Autodesk Fusion 360 part; units mm, degrees
sketch "Sketch1" plane through (0, 0, 0) normal (0, 0, 1) x (1, 0, 0)
  line L0 (-4.25, 7.25) -> (4.25, 7.25)
  line L1 (7.25, 4.25) -> (7.25, -4.25)
  line L2 (4.25, -7.25) -> (-4.25, -7.25)
  line L3 (-7.25, -4.25) -> (-7.25, 4.25)
  line L4 (-7.25, 7.25) -> (7.25, -7.25) construction
  line L5 (7.25, 7.25) -> (-7.25, -7.25) construction
  arc A0 (-4.25, 7.25) -> (-7.25, 4.25) centre (-4.25, 4.25) ccw
  arc A1 (-7.25, -4.25) -> (-4.25, -7.25) centre (-4.25, -4.25) ccw
  arc A2 (4.25, -7.25) -> (7.25, -4.25) centre (4.25, -4.25) ccw
  arc A3 (7.25, 4.25) -> (4.25, 7.25) centre (4.25, 4.25) ccw
  line L6 (10, 10) -> (-10, 10)
  line L7 (-15, 5) -> (-15, -5)
  line L8 (-10, -10) -> (10, -10)
  line L9 (15, -5) -> (15, 5)
  line L10 (15, 10) -> (-15, -10) construction
  line L11 (-15, 10) -> (15, -10) construction
  arc A4 (15, 5) -> (10, 10) centre (10, 5) ccw
  arc A5 (-10, 10) -> (-15, 5) centre (-10, 5) ccw
  arc A6 (-15, -5) -> (-10, -10) centre (-10, -5) ccw
  arc A7 (10, -10) -> (15, -5) centre (10, -5) ccw
  circle A8 centre (-12.5, 0) radius 1.6
  line L12 (0, 0) -> (0, 5.6259) construction
  circle A9 centre (12.5, 0) radius 1.6
  line L13 (-3, 4.4279) -> (-3, -3.4951) construction
  line L14 (6.15, 5.55) -> (-6.15, 5.55)
  line L15 (-6.15, 5.55) -> (-6.15, -5.55)
  line L16 (-6.15, -5.55) -> (6.15, -5.55)
  line L17 (6.15, -5.55) -> (6.15, 5.55)
  line L18 (6.15, 5.55) -> (-6.15, -5.55) construction
  line L19 (-6.15, 5.55) -> (6.15, -5.55) construction
  line L20 (-6.35, -5.75) -> (6.35, -5.75)
  line L21 (6.35, -5.75) -> (6.35, 5.75)
  line L22 (6.35, 5.75) -> (-6.35, 5.75)
  line L23 (-6.35, 5.75) -> (-6.35, -5.75)
  dimension "d1" = 14.5
  dimension "d2" = 14.5
  dimension "d3" = 3
  dimension "d4" = 30
  dimension "d5" = 20
  dimension "d6" = 5
  dimension "d7" = 3.2
  dimension "d17" = 12.5
  dimension "d21" = 12.3
  dimension "d22" = 11.1
  dimension "d23" = 0.2
extrude "Extrude1" add sketch "Sketch1" along normal blind 2.5 contours L0 L1 L2 L3 A0 A1 A2 A3 | L6 L7 L8 L9 A4 A5 A6 A7 | L20 L21 L22 L23
extrude "Extrude2" add sketch "Sketch1" against normal blind 11 contours L0 L1 L2 L3 A0 A1 A2 A3
Input: part model. Units: mm. Frame: model coordinates. A direction names the side the tool comes from. Give positions to 0.01 mm unless a question says otherwise; leave off trailing zeros. Order: outer loops, then holes, each group sorted by start corner. A loop starts at its lowest first (then second) coordinate and runs counter-clockwise, first axis right, second up.
Q1. Draft query along Y for faces 1 (the flat face through (0, 5.75, -5)), 2 (the flat face through (-6.35, 0, -5)), 3 (the cylindrical face through (13, 9, 1)), 4 (the flat face through (15, 0, 1)). Return one class per face: +Y half, -Y half, draft (parallel to the pull), parting line (faces both ways), or undercut.
Checked values:
face 1: undercut
face 2: undercut
face 3: +Y half
face 4: draft
Q2. Contact query for flat-ended pins moving along their axis: pin 1 Ø4 at (x, z) = (2, -4.5) entering from -Y; pin 2 Ø3.5 at (y, z) = (-1.5, -3) entering from -X; pin 3 Ø2 at (y, z) = (-1.5, -9.5) entering from +X. Output: stop coordinate, or through.
Checked values:
pin 1: stops at y = -7.25
pin 2: stops at x = -7.25
pin 3: stops at x = 7.25
Q3. Section A-A on y = 0. Output: boundary loops of the cut face in (x, z).
Checked values:
outline: (-15, 0) - (-14.1, 0) - (-14.1, 2.5) - (-15, 2.5) - close; (-10.9, 0) - (-7.25, 0) - (-7.25, -11) - (-6.35, -11) - (-6.35, 0) - (-6.15, 0) - (-6.15, 2.5) - (-10.9, 2.5) - close; (6.15, 0) - (6.35, 0) - (6.35, -11) - (7.25, -11) - (7.25, 0) - (10.9, 0) - (10.9, 2.5) - (6.15, 2.5) - close; (14.1, 0) - (15, 0) - (15, 2.5) - (14.1, 2.5) - close
Q4. Ray query, probe 1 along Y at (x, z) = (-3.5, -4.5); probe 2 along X at (y, z) = (0.25, -3.75); probe 3 along X at (y, z) = (2.75, 0.25). Return the intervals inside material, ascending.
Checked values:
probe 1: y = -7.25 to -5.75, 5.75 to 7.25
probe 2: x = -7.25 to -6.35, 6.35 to 7.25
probe 3: x = -15 to -6.15, 6.15 to 15
Q5. Set-up query: faces 5 (the flat face through (-7.25, 0, -5)), 6 (the cylindrical face through (6.39, 6.35, -5.42)), 7 (the cylindrical face through (6.35, -6.39, -5.42)). Return all of +Z, -Z, +X, -X, +Y, -Y with unobstructed straight access to the full face (end or side cutting, diameter ignored); none if empty.
Checked values:
face 5: -Z, -X, +Y, -Y
face 6: -Z, +X, +Y
face 7: -Z, +X, -Y
Q6. Section C-C on z = -8.25. Output: boundary loops of the cut face in (x, y), and give its area (3 significant figures).
Checked values:
outline: (-7.25, -4.25) arc R3 ccw to (-4.25, -7.25) - (4.25, -7.25) arc R3 ccw to (7.25, -4.25) - (7.25, 4.25) arc R3 ccw to (4.25, 7.25) - (-4.25, 7.25) arc R3 ccw to (-7.25, 4.25) - close; hole (-6.35, -5.75) - (6.35, -5.75) - (6.35, 5.75) - (-6.35, 5.75) - close
area: 56.5 mm2
Q7. Section B-B on y = -3.5. Output: boundary loops of the cut face in (x, z).
Checked values:
outline: (-15, 0) - (-7.25, 0) - (-7.25, -11) - (-6.35, -11) - (-6.35, 0) - (-6.15, 0) - (-6.15, 2.5) - (-15, 2.5) - close; (6.15, 0) - (6.35, 0) - (6.35, -11) - (7.25, -11) - (7.25, 0) - (15, 0) - (15, 2.5) - (6.15, 2.5) - close
Q8. Section D-D on x = 12.75. Output: boundary loops of the cut face in (y, z), and give its area (3 significant figures).
Checked values:
outline: (-9.18, 0) - (-1.58, 0) - (-1.58, 2.5) - (-9.18, 2.5) - close; (1.58, 0) - (9.18, 0) - (9.18, 2.5) - (1.58, 2.5) - close
area: 38.0 mm2
